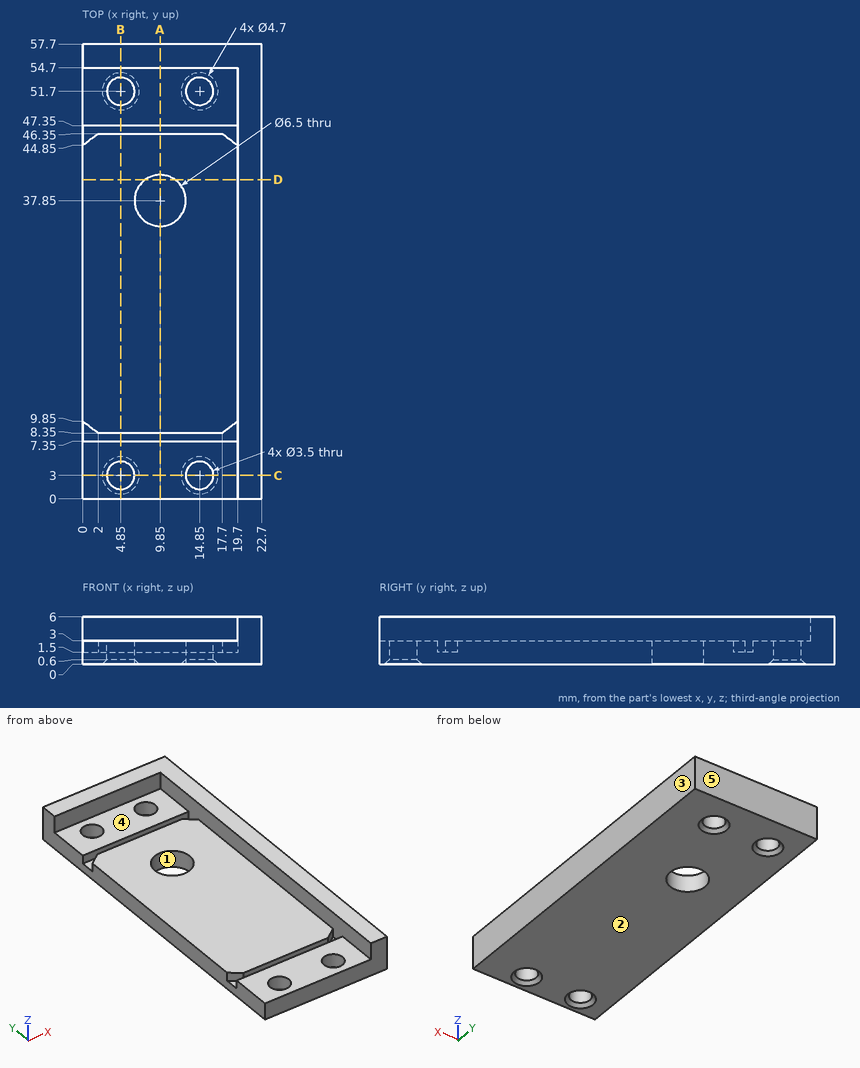
Check sheet for the drawn part. Datum: minimum x, y, z corner. Units: mm. A direction names the side the tool comes from. Coordinates: 2 decimals unless noted, no trailing zeros. Order: outer loops, then holes, each group sorted by start corner. A loop starts at its lowest first (then second) coordinate and runs counter-clockwise, first axis right, second up. Notation, with made-up numbers: (-2.5, 7) -> (19.5, 7) arc R23 ccw to (19.5, 23) -> close; hole circle Ø6 at (34.5, 59.5). An arc over 180 degrees is marked (long way). Write each question's results on one line, items separated by ' | '. Start each with the question number.
1) Set-up check for the marked faces 4 and 5: record each of +Z, -Z, +X, -X, +Y, -Y from which the full face is reachable in a straight line by a thin tool's end or side.
2) Section check C-C (y = 3). Enter the section's corners in (x, z), and give its area (3 significant figures).
3) Depth check by flat-ended pin: pin 1 (3.5 mm diameter, centred on x = 8, z = 4, fed in from -Y); pin 2 (3 mm diameter, centred on x = 4.85, y = 51.7, fed in from -Z); pin 3 (10 mm diameter, centred on x = 6, y = 32.5, fed in from +Z). Enter the tip coordinate at first touch or a pass-through.
4) Material ranges on line 1 along Y through (x, z) = (14.85, 1.25); line 2 along X through (y, z) = (51.7, 1.15); line 3 along Y through (x, z) = (9.85, 2), recorded low to high.
5) Section check D-D (y = 40.5). Enter the section's corners in (x, z), and give its area (3 significant figures).
6) Section check B-B (x = 4.85). Enter the section's corners in (y, z), and give its area (3 significant figures).
7) Draft check along X on the marked faces 1, 2 and 3. Enter one of: pulls with the +X half, pulls with the -X half, needs draft (parallel to the pull), parting line crosses it, or undercut.
8) Section check A-A (x = 9.85). Enter the section's corners in (y, z), and give its area (3 significant figures).
Checked values:
1) face 4: +Z, -X, -Y | face 5: +Z, -Z, +X, -X, +Y
2) outline: (0, 0) -> (2.5, 0) -> (3.1, 0.6) -> (3.1, 3) -> (0, 3) -> close; (6.6, 0.6) -> (7.2, 0) -> (12.5, 0) -> (13.1, 0.6) -> (13.1, 3) -> (6.6, 3) -> close; (16.6, 0.6) -> (17.2, 0) -> (22.7, 0) -> (22.7, 6) -> (19.7, 6) -> (19.7, 3) -> (16.6, 3) -> close | area: 55.4 mm²
3) pin 1: y = 0 | pin 2: through | pin 3: z = 3
4) line 1: 0 to 1.25, 4.75 to 49.95, 53.45 to 57.7 | line 2: 0 to 3.1, 6.6 to 13.1, 16.6 to 22.7 | line 3: 0 to 7.35, 8.35 to 34.6, 41.1 to 46.35, 47.35 to 57.7
5) outline: (0, 0) -> (7.97, 0) -> (7.97, 3) -> (0, 3) -> close; (11.73, 0) -> (22.7, 0) -> (22.7, 6) -> (19.7, 6) -> (19.7, 3) -> (11.73, 3) -> close | area: 65.8 mm²
6) outline: (0, 0) -> (0.65, 0) -> (1.25, 0.6) -> (1.25, 3) -> (0, 3) -> close; (4.75, 0.6) -> (5.35, 0) -> (49.35, 0) -> (49.95, 0.6) -> (49.95, 3) -> (47.35, 3) -> (47.35, 1.5) -> (46.35, 1.5) -> (46.35, 3) -> (8.35, 3) -> (8.35, 1.5) -> (7.35, 1.5) -> (7.35, 3) -> (4.75, 3) -> close; (53.45, 0.6) -> (54.05, 0) -> (57.7, 0) -> (57.7, 6) -> (54.7, 6) -> (54.7, 3) -> (53.45, 3) -> close | area: 157 mm²
7) face 1: undercut | face 2: needs draft | face 3: pulls with the +X half
8) outline: (0, 0) -> (34.6, 0) -> (34.6, 3) -> (8.35, 3) -> (8.35, 1.5) -> (7.35, 1.5) -> (7.35, 3) -> (0, 3) -> close; (41.1, 0) -> (57.7, 0) -> (57.7, 6) -> (54.7, 6) -> (54.7, 3) -> (47.35, 3) -> (47.35, 1.5) -> (46.35, 1.5) -> (46.35, 3) -> (41.1, 3) -> close | area: 160 mm²
